Design review of the part built by this model. Coordinates are the model's own, in mm. A direction names the side the tool comes from. Coordinates: 2 decimals unless noted, no trailing zeros. Loops run counter-clockwise (first coordinate to the right, second up) from the corner with the lowest first, then second, coordinate; pieces in that order, holes last. Notation, with made-up numbers: M 38,48 L 82,48 A16 ccw 82,73 Z; hole C 61,-22 d5. An arc over 180 degrees is marked long. Answer as a JSON object with one key per item and string values. Group by question number.
1. Draft analysis for pull direction Y (two halves, no side actions). For faces 6 (the flat face through (-3, 13, -10)), 7 (the flat face through (0, 18.5, -11)), 8 (the cylindrical face through (-8.4, 1.2, -5.6)), 9 (the flat face through (0, 2.5, -9.4)), state which applies: +Y half, -Y half, draft (parallel to the pull), parting line (faces both ways), or undercut.
2. Machinability: for faces 1 (the cylindrical face through (6.074, 1.232, -0.044)), 2 (the flat face through (1.5, 9.9, -10)), 3 (the flat face through (-7.258, 1.232, -9.726)), 4 (the flat face through (-4, 10, -10)), 5 (the cylindrical face through (0.26, 1.23, -7.83)), which of the approach directions +Z, -Z, +X, -X, +Y, -Y give a long, thin tool a straight path to every point of the face, cutting with its end or side? Answer none if there is none.
3. To check wall thickness, follow probe 1 along X at (y, z) = (0.75, 0) (3 decimals); probe 2 along Z at (x, y) = (0, 0.65); probe 3 along Y at (x, z) = (-6.75, -1.25). State the ranges of each line that lie inside material, in increasing order.
4. Consider section A-A (y = 12.5). State the section outline as (x, z) points.
5. Consider section D-D (x = 9.4). State the section outline as (y, z) points.
6. Consider section B-B (x = -4.5). State the section outline as (y, z) points.
7. Consider section C-C (z = -0.5). State the section outline as (x, y) points.
8. Insertion check: pin 1 (2.5 mm diameter, centred on y = 12, z = -9.5, fed in from +X); pin 2 (1.2 mm diameter, centred on y = 13.5, z = -10.5, fed in from -X); pin 3 (1.8 mm diameter, centred on x = -1, y = 13, fed in from +Z); pin 4 (4 mm diameter, centred on x = 7.5, y = 14.5, fed in from +Z). Each pin has a flat end and moves straight along its axis. Give the tip position at first contact, or say it passes through.
Autodesk Inventor part; units mm, degrees
ref_plane "Work Plane1" through (0, 18.5, -9) normal (0, 0, 1) x (1, 0, 0)
ref_plane "YZ Plane" through (0, 0, 0) normal (1, 0, 0) x (0, 1, 0)
ref_plane "XZ Plane" through (0, 0, 0) normal (0, 1, 0) x (-1, 0, 0)
sketch "sk_base" plane through (0, 0, 0) normal (0, 1, 0) x (-1, 0, 0)
  line L0 (16.4021, 0) -> (-16.8737, 0)
  line L1 (0, -22.2) -> (0, 14.2)
  circle A0 centre (0, 0) radius 8.8 construction
  circle A1 centre (0, -9) radius 1.2
  circle A2 centre (5.075, 0) radius 1
  circle A3 centre (-5.075, 0) radius 1
  circle A4 centre (0, 0) radius 3.4
  line L2 (9.4, -5.5883) -> (-9.4, 5.5883) construction
  circle A5 centre (9.4, -5.5883) radius 1 construction
  circle A6 centre (-9.4, 5.5883) radius 1 construction
  circle A7 centre (0, 0) radius 9 construction
  circle A8 centre (0, -9) radius 8 construction
  circle A9 centre (9.4, -5.5883) radius 2 construction
  circle A10 centre (-9.4, 5.5883) radius 2 construction
  line L3 (-8.6663, 7.4488) -> (8.9868, 0.4877)
  line L4 (8.9868, 0.4877) -> (11.2402, -4.8048)
  line L5 (4, -8.0623) -> (4, -12.2) construction
  line L6 (4, -12.2) -> (-4, -12.2)
  line L7 (-4, -12.2) -> (-4, -8.0623) construction
  line L8 (4, -9) -> (-4, -9) construction
  line L9 (4, -12.2) -> (10.6095, -7.1811)
  arc A11 (10.6095, -7.1811) -> (11.2402, -4.8048) centre (9.4, -5.5883) ccw
  line L10 (-11.2402, 4.8048) -> (-6.8151, -5.5883)
  line L11 (9.4, -5.5883) -> (-6.8151, -5.5883) construction
  arc A12 (-8.6663, 7.4488) -> (-11.2402, 4.8048) centre (-9.4, 5.5883) ccw
  line L12 (7.6889, 3.536) -> (-8.9324, 7.5328)
  line L13 (-4, -12.2) -> (-6.8151, -5.5883)
  line L14 (7.6889, 3.536) -> (8.9868, 0.4877)
  circle A13 centre (9.4, -5.5883) radius 1
  circle A14 centre (-9.4, 5.5883) radius 1
  dimension "d0" = 17.6
  dimension "d1" = 10.15
  dimension "d2" = 2
  dimension "d3" = 6.8
  dimension "servo_dowel_diameter" = 2.4
  dimension "servo_distance_gearcenters" = 9
  dimension "d7" = 18
  dimension "d8" = 16
  dimension "d10" = 4
  dimension "d11" = 3.2
  dimension "d12" = 8
  dimension "d13" = 8
  dimension "d16" = 9.4
  dimension "m2_screw_selfthreading_hole_diam" = 2
extrude "ext_front" add sketch "sk_base" along normal blind 2.5 contours L4 A11 L9 L6 L1 A1 A4 L0 A2 | L0 A2 A4 L1 L3 L4 | L3 L1 L12 L14 | L3 A12 L12 L1 | L1 A4 L0 A3 L10 A12 L3 | L1 A1 L6 L13 L10 L0 A3 A4
sketch "Sketch2" plane through (0, 2.5, 0) normal (0, 1, 0) x (1, 0, 0)
  line L0 (-4, 8.0623) -> (-4, 12.2) construction
  line L1 (-4, 9) -> (4, 9) construction
  line L2 (4, 12.2) -> (4, 8.0623) construction
  circle A0 centre (0, 0) radius 9 construction
  line L3 (4, 12.2) -> (-4, 12.2)
  line L4 (-4, 12.2) -> (-4, 9)
  line L5 (-4, 9) -> (4, 9)
  line L6 (4, 9) -> (4, 12.2)
  arc A1 (4, 8.0623) -> (-4, 8.0623) centre (0, 0) ccw
  line L7 (4, 8.0623) -> (4, 9)
  line L8 (-4, 8.0623) -> (-4, 9)
extrude "ext_backsupport" add sketch "Sketch2" along normal blind 16
ref_plane "Work Plane1" through (0, 18.5, -9) normal (0, 0, 1) x (1, 0, 0)
sketch "sk_mounthole" plane through (0, 18.5, -9) normal (0, 0, 1) x (1, 0, 0)
  line L0 (-1.1973, -16) -> (1.1973, -16)
  line L1 (0, -22.2) -> (0, 3.7)
  circle A0 centre (0, -6) radius 1.5
  line L2 (0, -2.5359) -> (-3, -4.2679)
  line L3 (-3, -4.2679) -> (-3, -7.7321)
  line L4 (-3, -7.7321) -> (0, -9.4641)
  line L5 (0, -9.4641) -> (3, -7.7321)
  line L6 (3, -7.7321) -> (3, -4.2679)
  line L7 (3, -4.2679) -> (0, -2.5359)
  line L8 (-3, -6) -> (3, -6) construction
  point P0 (0, -18.5)
  dimension "m3_screw_max_diam" = 3
  dimension "d23" = 120
  dimension "d24" = 10
extrude "ext_mounthole" cut sketch "sk_mounthole" along normal through all both and the other way through all contours A0 L1 | L1 A0
extrude "ext_mountnut" cut sketch "sk_mounthole" along normal blind 10 and the other way blind 2.4
equation "\"d2\" = screw_m2_bore_selfthreading"
equation "\"servo_dowel_diameter\" = general_dowel_diameter"
equation "\"m2_screw_selfthreading_hole_diam\" = screw_m2_bore_selfthreading"
properties part number "empty"
Findings below:
{
 "1": {"face 6": "undercut", "face 7": "+Y half", "face 8": "draft", "face 9": "-Y half"},
 "2": {"face 1": "+Y, -Y", "face 2": "+Z", "face 3": "-Z, -X, +Y, -Y", "face 4": "+Z, -Z, -X, +Y", "face 5": "-Y"},
 "3": {"probe 1": "x = -9.194 to -6.075, -4.075 to -3.4, 3.4 to 4.075, 6.075 to 9.194", "probe 2": "z = -12.2 to -10.2, -7.8 to -3.4, 3.4 to 5.38", "probe 3": "y = 0 to 2.5"},
 "4": {"outline": "M -4,-12.2 L -1.5,-12.2 L -1.5,-11.4 L -3,-11.4 L -3,-8.49 A9 cw -4,-8.06 Z; M 1.5,-12.2 L 4,-12.2 L 4,-8.06 A9 cw 3,-8.49 L 3,-11.4 L 1.5,-11.4 Z"},
 "5": {"outline": "M 0,0.48 L 2.5,0.48 L 2.5,4.59 L 0,4.59 Z; M 0,6.59 L 2.5,6.59 L 2.5,7.59 L 0,7.59 Z"},
 "6": {"outline": "M 0,-11.82 L 2.5,-11.82 L 2.5,-0.82 L 0,-0.82 Z; M 0,0.82 L 2.5,0.82 L 2.5,4.3 L 0,4.3 Z"},
 "7": {"outline": "M -9.41,0 L -5.94,0 L -5.94,2.5 L -9.41,2.5 Z; M -4.21,0 L -3.36,0 L -3.36,2.5 L -4.21,2.5 Z; M 3.36,0 L 4.21,0 L 4.21,2.5 L 3.36,2.5 Z; M 5.94,0 L 8.98,0 L 8.98,2.5 L 5.94,2.5 Z"},
 "8": {"pin 1": "stops at x = 4", "pin 2": "stops at x = -4", "pin 3": "stops at z = -11.4", "pin 4": "passes through"}
}
